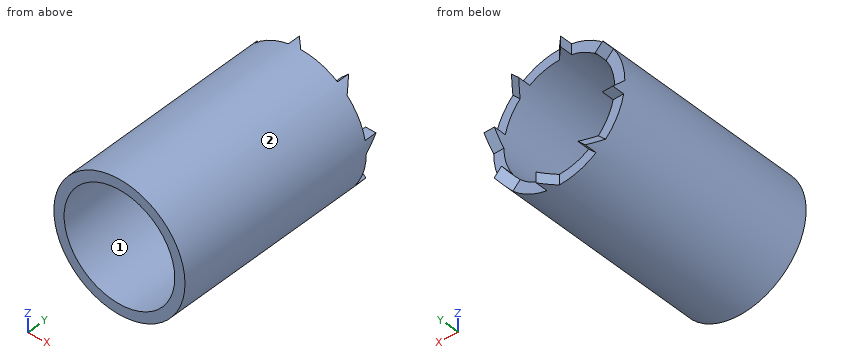
from build123d import *

# Parameters (mm, degrees)
SKETCH1_R           = 8.25
SKETCH1_R_2         = 6.75
BOSS_EXTRUDE1_DEPTH = 25
SKETCH2_W           = 1.5
SKETCH2_H           = 1.75
SKETCH2_W_2         = 1.75
SKETCH2_H_2         = 1.5
SKETCH2_H_3         = 1.499622071
BOSS_EXTRUDE2_DEPTH = 1.5
CUT_EXTRUDE1_DEPTH  = 2.5
CUT_EXTRUDE2_DEPTH  = 2.5
CUT_EXTRUDE3_DEPTH  = 2.5
CUT_EXTRUDE4_DEPTH  = 2.5
SKETCH9_R           = 6.625
CUT_EXTRUDE7_DEPTH  = 2.5
CUT_EXTRUDE10_DEPTH = 20.91726189
CUT_EXTRUDE11_DEPTH = 20.91726189
CUT_EXTRUDE12_DEPTH = 20.91726189
CUT_EXTRUDE13_DEPTH = 20.91726189
SKETCH15_R          = 10.332276799
SKETCH15_R_2        = 8
CUT_EXTRUDE14_DEPTH = 35
SKETCH16_R          = 6.75
CUT_EXTRUDE15_DEPTH = 40


with BuildPart() as part:
    # Sketch1 → Boss-Extrude1 (new body)
    with BuildSketch(Plane(origin=(0, 0, 0), x_dir=(1, 0, 0), z_dir=(0, 1, 0))):
        Circle(SKETCH1_R)
        Circle(SKETCH1_R_2, mode=Mode.SUBTRACT)
    extrude(amount=BOSS_EXTRUDE1_DEPTH)

    # Sketch2 → Boss-Extrude2 (add)
    with BuildSketch(Plane(origin=(0, 25, 0), x_dir=(1, 0, 0), z_dir=(0, 1, 0))):
        with Locations((0.75, 7.375)):
            Rectangle(SKETCH2_W, SKETCH2_H)
        with Locations((7.375, -0.75)):
            Rectangle(SKETCH2_W_2, SKETCH2_H_2)
        with Locations((-0.75, -7.375)):
            Rectangle(SKETCH2_W, SKETCH2_H)
        with Locations((-7.375, 0.749811036)):
            Rectangle(SKETCH2_W_2, SKETCH2_H_3)
        Polygon((-5.833630945, 5.833630945), (-4.772970773, 6.894291117), (-3.535533906, 5.656854249), (-4.596194078, 4.596194078), align=None)
        Polygon((5.833630945, 5.833630945), (6.894291117, 4.772970773), (5.656854249, 3.535533906), (4.596194078, 4.596194078), align=None)
        Polygon((5.833630945, -5.833630945), (4.772970773, -6.894291117), (3.535533906, -5.656854249), (4.596194078, -4.596194078), align=None)
        Polygon((-5.833630945, -5.833630945), (-6.894291117, -4.772970773), (-5.656854249, -3.535533906), (-4.596194078, -4.596194078), align=None)
    extrude(amount=BOSS_EXTRUDE2_DEPTH)

    # Sketch5 → Cut-Extrude1 (cut)
    with BuildSketch(Plane.XY.offset(8.25)):
        Polygon((-1.5, 26.5), (0, 25), (0, 26.5), align=None)
    extrude(amount=-CUT_EXTRUDE1_DEPTH, mode=Mode.SUBTRACT)

    # Sketch6 → Cut-Extrude2 (cut)
    with BuildSketch(Plane.ZY.offset(8.25)):
        Polygon((0, 26.5), (-1.499622071, 26.5), (0, 25), align=None)
    extrude(amount=-CUT_EXTRUDE2_DEPTH, mode=Mode.SUBTRACT)

    # Sketch7 → Cut-Extrude3 (cut)
    with BuildSketch(Plane(origin=(0, 0, -8.25), x_dir=(-1, 0, 0), z_dir=(0, 0, -1))):
        Polygon((-1.5, 26.5), (0, 26.5), (0, 25), align=None)
    extrude(amount=-CUT_EXTRUDE3_DEPTH, mode=Mode.SUBTRACT)

    # Sketch8 → Cut-Extrude4 (cut)
    with BuildSketch(Plane(origin=(8.25, 0, 0), x_dir=(0, 0, -1), z_dir=(1, 0, 0))):
        Polygon((0, 26.5), (-1.5, 26.5), (0, 25), align=None)
    extrude(amount=-CUT_EXTRUDE4_DEPTH, mode=Mode.SUBTRACT)

    # Sketch9 → Cut-Extrude7 (cut)
    with BuildSketch(Plane(origin=(0, 25, 0), x_dir=(1, 0, 0), z_dir=(0, 1, 0))):
        Circle(SKETCH9_R)
    extrude(amount=CUT_EXTRUDE7_DEPTH, mode=Mode.SUBTRACT)

    # Sketch11 → Cut-Extrude10 (cut, through all)
    with BuildSketch(Plane(origin=(-5.833630945, 0, 5.833630945), x_dir=(0.707106781, 0, 0.707106781), z_dir=(-0.707106781, 0, 0.707106781))):
        Polygon((0, 25), (-1.5, 26.5), (0, 26.5), align=None)
    extrude(amount=-CUT_EXTRUDE10_DEPTH, mode=Mode.SUBTRACT)

    # Sketch12 → Cut-Extrude11 (cut, through all)
    with BuildSketch(Plane(origin=(-5.833630945, 0, -5.833630945), x_dir=(-0.707106781, 0, 0.707106781), z_dir=(-0.707106781, 0, -0.707106781))):
        Polygon((0, 25), (-1.5, 26.5), (0, 26.5), align=None)
    extrude(amount=-CUT_EXTRUDE11_DEPTH, mode=Mode.SUBTRACT)

    # Sketch13 → Cut-Extrude12 (cut, through all)
    with BuildSketch(Plane(origin=(5.833630945, 0, -5.833630945), x_dir=(-0.707106781, 0, -0.707106781), z_dir=(0.707106781, 0, -0.707106781))):
        Polygon((0, 25), (-1.5, 26.5), (0, 26.5), align=None)
    extrude(amount=-CUT_EXTRUDE12_DEPTH, mode=Mode.SUBTRACT)

    # Sketch14 → Cut-Extrude13 (cut, through all)
    with BuildSketch(Plane(origin=(5.833630945, 0, 5.833630945), x_dir=(0.707106781, 0, -0.707106781), z_dir=(0.707106781, 0, 0.707106781))):
        Polygon((0, 25), (-1.5, 26.5), (0, 26.5), align=None)
    extrude(amount=-CUT_EXTRUDE13_DEPTH, mode=Mode.SUBTRACT)

    # Sketch15 → Cut-Extrude14 (cut)
    with BuildSketch(Plane.XZ):
        Circle(SKETCH15_R)
        Circle(SKETCH15_R_2, mode=Mode.SUBTRACT)
    extrude(amount=-CUT_EXTRUDE14_DEPTH, mode=Mode.SUBTRACT)

    # Sketch16 → Cut-Extrude15 (cut)
    with BuildSketch(Plane(origin=(0, 0, 0), x_dir=(1, 0, 0), z_dir=(0, 1, 0))):
        Circle(SKETCH16_R)
    extrude(amount=CUT_EXTRUDE15_DEPTH, mode=Mode.SUBTRACT)


solid = part.part
Build history of the part. All positions in model axes, mm. Face numbers are marked on the shaded views. Round coordinates to 2 decimals unless told otherwise and drop trailing zeros. Write each loop counter-clockwise with the first axis right and the second up, starting at its lowest first coordinate (ties: lowest second). Pieces come first, ordered by that corner, then holes. Notation, with made-up numbers: (63, -5) -> (75, -5) arc R12 cw to (75, 0) -> close; hole circle Ø10 at (-35.5, 34.25). An arc over 180 degrees is marked (long way). Use one line per item in the form item = value.
Q1. Band-saw the part on A-A, the plane z = -2.5. Write the cut outline in (x, y).
Conclusion:
outline = (-7.6, 0) -> (-6.27, 0) -> (-6.27, 25) -> (-7.6, 25) -> close; (6.27, 0) -> (7.6, 0) -> (7.6, 25) -> (6.27, 25) -> close
Q2. Band-saw the part on C-C, the plane y = 8.5. Write the cut outline in (x, z).
Conclusion:
outline = circle Ø16 at (0, 0); hole circle Ø13.5 at (0, 0)
Q3. Band-saw the part on B-B, the plane x = 0.5. Write the cut outline in (y, z), then the cut area to 3 significant figures.
Conclusion:
outline = (0, -7.98) -> (25.5, -7.98) -> (25.5, -6.73) -> (0, -6.73) -> close; (0, 6.73) -> (25, 6.73) -> (25, 7.98) -> (0, 7.98) -> close
area = 63.3 mm²
Q4. Two-plate mould, pull along X, no slides. Class the marked faces 1 and 2: released by +X, released by -X, zero draft, split by the parting line, or undercut.
Conclusion:
face_1 = undercut
face_2 = split by the parting line
Q5. Drill centre lines: L1, parallel to Z at x = 0, y = 12; L2, parallel to X at y = 17.5, z = 1.5. Where is each one in solid material? Low to high.
Conclusion:
L1 = -8 to -6.75, 6.75 to 8
L2 = -7.86 to -6.58, 6.58 to 7.86
Q6. Band-saw the part on D-D, the plane z = -5.25. Write the cut outline in (x, y), then the cut area to 3 significant figures.
Conclusion:
outline = (-6.04, 0) -> (-4.24, 0) -> (-4.24, 25.71) -> (-5.25, 25) -> (-6.04, 25) -> close; (4.24, 0) -> (6.04, 0) -> (6.04, 25.56) -> (5.25, 25) -> (4.24, 25) -> close
area = 90.3 mm²
Q7. Drop flat-ended pins along their axis: P1, Ø1.1, axis at x = -6.5, z = 2.5, coming from the +Y side; P2, Ø1, axis at x = 3, y = 23, coming from the -Z side; P3, Ø1, axis at x = -3.5, y = 3.5, coming from the +Z side. Give the stop position or say it passes through.
Conclusion:
P1 = 25
P2 = -7.6
P3 = 7.42
